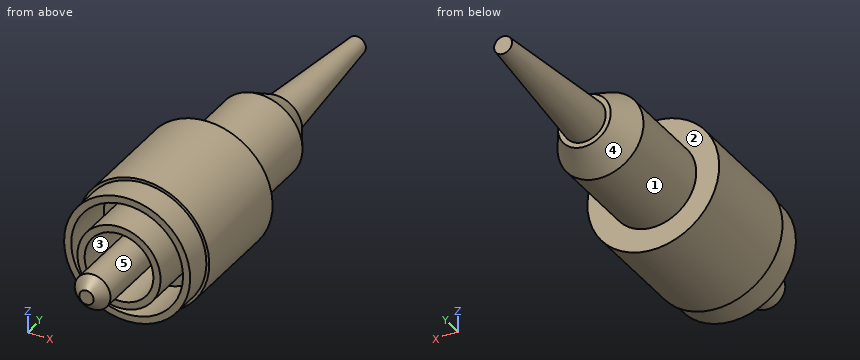
from build123d import *

# Parameters (mm, degrees)
SKETCH_1_R          = 4.6
EXTRUDE_1_DEPTH     = 9.8
SKETCH_2_R          = 4.6
SKETCH_2_R_2        = 4.4
CUT_EXTRUDE_1_DEPTH = 2
SKETCH_3_R          = 3.9
SKETCH_3_R_2        = 2.9
CUT_EXTRUDE_2_DEPTH = 4
SKETCH_4_R          = 2.4
CUT_EXTRUDE_3_DEPTH = 5
SKETCH_5_R          = 1.25
EXTRUDE_4_DEPTH     = 10
CHAMFER_1_SIZE      = 0.75
EXTRUDE_START       = 1
SKETCH_6_R          = 2.9
SKETCH_6_R_2        = 2.4
EXTRUDE_5_DEPTH     = 1
SKETCH_7_R          = 3
EXTRUDE_6_DEPTH     = 8.5
CHAMFER_2_SIZE      = 2
CHAMFER_2_SIZE2     = 1.154700538
SKETCH_8_R          = 1.5
EXTRUDE_7_DEPTH     = 10
CHAMFER_3_SIZE      = 10
CHAMFER_3_SIZE_2    = 0.874886635


with BuildPart() as part:
    # 草图1 → 拉伸1 (new body)
    with BuildSketch(Plane(origin=(0, 0, 0), x_dir=(1, 0, 0), z_dir=(0, 1, 0))):
        with Locations(Location((0, 0, 0), (0, 0, 270))):
            Circle(SKETCH_1_R)
    extrude(amount=EXTRUDE_1_DEPTH)

    # 草图2 → 切除-拉伸1 (cut)
    with BuildSketch(Plane.XZ):
        with Locations(Location((0, 0, 0), (0, 0, 270))):
            Circle(SKETCH_2_R)
        with Locations(Location((0, 0, 0), (0, 0, 270))):
            Circle(SKETCH_2_R_2, mode=Mode.SUBTRACT)
    extrude(amount=-CUT_EXTRUDE_1_DEPTH, mode=Mode.SUBTRACT)

    # 草图3 → 切除-拉伸2 (cut)
    with BuildSketch(Plane.XZ):
        with Locations(Location((0, 0, 0), (0, 0, 270))):
            Circle(SKETCH_3_R)
        with Locations(Location((0, 0, 0), (0, 0, 270))):
            Circle(SKETCH_3_R_2, mode=Mode.SUBTRACT)
    extrude(amount=-CUT_EXTRUDE_2_DEPTH, mode=Mode.SUBTRACT)

    # 草图4 → 切除-拉伸3 (cut)
    with BuildSketch(Plane.XZ):
        with Locations(Location((0, 0, 0), (0, 0, 270))):
            Circle(SKETCH_4_R)
    extrude(amount=-CUT_EXTRUDE_3_DEPTH, mode=Mode.SUBTRACT)

    # 草图5 → 拉伸4 (add)
    with BuildSketch(Plane.XZ.offset(-5)):
        with Locations(Location((0, 0, 0), (0, 0, 270))):
            Circle(SKETCH_5_R)
    extrude(amount=EXTRUDE_4_DEPTH)

    # 倒角1
    chamfer_1_edges = [part.edges().sort_by_distance(p)[0] for p in [
        (0, -5, 1.25),
    ]]
    chamfer(chamfer_1_edges, length=CHAMFER_1_SIZE)

    # 草图6 → 拉伸5 (add)
    with BuildSketch(Plane.XZ.offset(EXTRUDE_START)):
        with Locations(Location((0, 0, 0), (0, 0, 270))):
            Circle(SKETCH_6_R)
        with Locations(Location((0, 0, 0), (0, 0, 270))):
            Circle(SKETCH_6_R_2, mode=Mode.SUBTRACT)
    extrude(amount=-EXTRUDE_5_DEPTH)

    # 草图7 → 拉伸6 (add)
    with BuildSketch(Plane(origin=(0, 9.8, 0), x_dir=(-1, 0, 0), z_dir=(0, 1, 0))):
        with Locations(Location((0, 0, 0), (0, 0, 90))):
            Circle(SKETCH_7_R)
    extrude(amount=EXTRUDE_6_DEPTH)

    # 倒角2
    chamfer_2_edges = [part.edges().sort_by_distance(p)[0] for p in [
        (0, 18.3, -3),
    ]]
    chamfer_2_side = [part.faces().sort_by_distance(p)[0] for p in [
        (0, 14.05, -3),
    ]]
    chamfer(chamfer_2_edges, length=CHAMFER_2_SIZE, length2=CHAMFER_2_SIZE2, reference=chamfer_2_side[0])

    # 草图8 → 拉伸7 (add)
    with BuildSketch(Plane(origin=(0, 18.3, 0), x_dir=(-1, 0, 0), z_dir=(0, 1, 0))):
        with Locations(Location((0, 0, 0), (0, 0, 90))):
            Circle(SKETCH_8_R)
    extrude(amount=EXTRUDE_7_DEPTH)

    # 倒角3
    # the kernel refuses this chamfer: 10, 0.874886635 mm, written as the material it takes off along each edge
    with BuildSketch(Plane(origin=(0, 28.3, 0), x_dir=(0, 0, 1), z_dir=(-1, 0, 0))) as chamfer_3_piece_1_section:
        Polygon((1.5, -CHAMFER_3_SIZE), (1.5 - CHAMFER_3_SIZE_2, 0), (1.5, 0), align=None)
    chamfer_3_piece_1 = revolve(axis=Axis((0, 28.3, 0), (0, 1, 0)), mode=Mode.PRIVATE)
    chamfer_3_piece_1 = split(chamfer_3_piece_1, bisect_by=Plane(origin=(0, 18.3, -1.083102127), z_dir=(0, 1, 0)), keep=Keep.TOP, mode=Mode.PRIVATE)
    add(chamfer_3_piece_1, mode=Mode.SUBTRACT)


solid = part.part
CAD build for the part. Positions are in the model's coordinates, mm. Face numbers are marked on the shaded views. A direction names the side the tool comes from. Give positions to 0.01 mm unless a question says otherwise; leave off trailing zeros. Loops run counter-clockwise (first coordinate to the right, second up) from the corner with the lowest first, then second, coordinate; pieces in that order, holes last. Notation, with made-up numbers: M 16.25,38 L 58.25,38 A18 cw 58.25,54 Z; hole C 57.25,49 d11. An arc over 180 degrees is marked long. Write each question's results on one line, items separated by ' | '.
Q1. Band-saw the part on A-A on y = 0.5. Write the cut outline in (x, z), and give its area (3 significant figures).
Geometry check:
outline: C 0,0 d8.8; C 0,0 d5.8; C 0,0 d2.5; hole C 0,0 d7.8; hole C 0,0 d4.8 | area: 26.3 mm²
Q2. Band-saw the part on B-B on y = 16. Write the cut outline in (x, z).
Geometry check:
outline: C 0,0 d6
Q3. Probe probe 1 along X at (y, z) = (0.4, 0); probe 2 along X at (y, z) = (2.8, 0); probe 3 along Y at (x, z) = (-3.5, 1.25). List the from-to ranges inside material, lowest first.
Geometry check:
probe 1: x = -4.4 to -3.9, -2.9 to -2.4, -1.25 to 1.25, 2.4 to 2.9, 3.9 to 4.4 | probe 2: x = -4.6 to -3.9, -2.9 to -2.4, -1.25 to 1.25, 2.4 to 2.9, 3.9 to 4.6 | probe 3: y = 4 to 9.8
Q4. Band-saw the part on D-D on y = 9.5. Write the cut outline in (x, z), and give its area (3 significant figures).
Geometry check:
outline: C 0,0 d9.2 | area: 66.5 mm²
Q5. Band-saw the part on C-C on z = 3.5. Write the cut outline in (x, y).
Geometry check:
outline: M -2.98,2 L -2.67,2 L -2.67,0 L -1.72,0 L -1.72,4 L 1.72,4 L 1.72,0 L 2.67,0 L 2.67,2 L 2.98,2 L 2.98,9.8 L -2.98,9.8 Z
Q6. Flat gauge pins, fed straight in: P1, Ø5, axis at x = -3, z = -1, coming from the -Y side; P2, Ø1, axis at y = 14, z = 0.5, coming from the +X side; P3, Ø2, axis at x = 2.5, y = 9.5, coming from the -Z side. Where does each tip first touch, or does it go through?
Geometry check:
P1: stops at y = -4.84 | P2: stops at x = 3 | P3: stops at z = -4.35
Q7. Mould opens along Z. For the marked faces 1, 2 and 3 say: pulls with the +Z half, pulls with the -Z half, needs draft (parallel to the pull), parting line crosses it, or undercut.
Geometry check:
face 1: parting line crosses it | face 2: needs draft | face 3: undercut
Q8. Which spindle directions (+Z, -Z, +X, -X, +Y, -Y) get a long thin tool onto all of the face, cutting with end or side? Do the marked faces 4 and 5. Say none if no direction does.
Geometry check:
face 4: +Y | face 5: -Y
